Read the model definition and answer for the solid it produces. Units are mm, in the model's axes. Coordinates: 2 decimals unless noted, no trailing zeros. Loops run counter-clockwise (first coordinate to the right, second up) from the corner with the lowest first, then second, coordinate; pieces in that order, holes last. Notation, with made-up numbers: (28.5, 2.5) - (47.5, 2.5) arc R23 cw to (47.5, 16.5) - close; hole circle Ø11 at (-14.75, 63). An arc over 180 degrees is marked (long way). Use one line per item in the form item = value. Start each with the question number.
1) The mould has two halves that part along X. Classify faces 1 (the face through (0, 0, 0)), 2 (the face through (3, -6, 20)), 3 (the face through (12.932, 5.362, 10.114)): released by +X, released by -X, zero draft, split by the parting line, or undercut.
2) Consider line 1 (Y direction, x = 0, z = 5); line 2 (Y direction, x = 4, z = 17.75). Determine where each line is inside the solid, lowest interval first.
3) Each of these flat-tipped pins is pushed along its axis until it touches: P1, Ø5, axis at y = -3, z = 3, coming from the -X side; P2, Ø12, axis at x = -9.5, z = 9.5, coming from the +Y side; P3, Ø6, axis at x = 0.5, y = 0.5, coming from the +Z side. Where does it stop, or does it pass through?
4) A cutting plane is placed at A-A (z = 18). Give the vertices of the cut face in (x, y).
Autodesk Inventor part; units mm, degrees
ref_plane "YZ Plane" through (0, 0, 0) normal (1, 0, 0) x (0, 1, 0)
ref_plane "XZ Plane" through (0, 0, 0) normal (0, 1, 0) x (-1, 0, 0)
ref_plane "XY Plane" through (0, 0, 0) normal (0, 0, 1) x (1, 0, 0)
sketch "Szkic1" plane through (0, 0, 0) normal (0, 0, 1) x (1, 0, 0)
  circle A0 centre (0, 0) radius 14
  dimension "d0" = 28
extrude "Wyciągnięcie proste1" add sketch "Szkic1" along normal blind 20
shell "Skorupa1" thickness 8 removed faces 2 at (0.5625, 1.5565, 0) at (0.5625, 1.5565, 20)
sketch "Szkic2" plane through (0, 0, 0) normal (0, 1, 0) x (-1, 0, 0)
  line L0 (-14, 0) -> (14, 0) construction
  line L1 (0, 0) -> (16, 0)
  line L2 (0, 0) -> (0, -3)
  arc A0 (0, -3) -> (16, 0) centre (0, 41.1667) ccw
  dimension "d4" = 16
  dimension "d5" = 3
revolve "Obrót1" add sketch "Szkic2" angle 360 about axis through (0, 0, 0) along (0, 0, -1)
fillet "Zaokrąglenie1" radius 0.5 1 edges at (-14, 0, 0)
thread "Gwint1"
properties part number "Zaślepka_do_widelca" material "Polietylen o dużej gęstości"
Found:
q1.face_1 = undercut
q1.face_2 = zero draft
q1.face_3 = split by the parting line
q2.line_1 = -14 to -6, 6 to 14
q2.line_2 = -13.42 to -4.47, 4.47 to 13.42
q3.P1 = -13.99
q3.P2 = 13.56
q3.P3 = 0
q4.outline = circle Ø28 at (0, 0); hole circle Ø12 at (0, 0)
